Part model, mm, in its own coordinate system. Round coordinates to 2 decimals unless told otherwise and drop trailing zeros. Write each loop counter-clockwise with the first axis right and the second up, starting at its lowest first coordinate (ties: lowest second). Pieces come first, ordered by that corner, then holes. Notation, with made-up numbers: M 20.5,76.25 L 60.5,76.25 A21 cw 60.5,98.25 Z; hole C 14,17 d1. An arc over 180 degrees is marked long. One line per question, with ' | ' between items. Start each with the question number.
1) Saw through at B-B (z = 77.5). List the corners of the cut face in (x, y).
2) Drop flat-ended pins along their axis: pin 1 Ø12 at (x, y) = (9, -44.5) entering from -Z; pin 2 Ø10 at (y, z) = (-64, 26.5) entering from -X; pin 3 Ø4 at (x, y) = (9.5, -52.5) entering from +Z; pin 4 Ø1 at (x, y) = (21.5, -11.5) entering from +Z. Give the stop position or say it passes through.
3) Saw through at C-C (x = -17). List the corners of the cut face in (y, z), plus the area to 3 significant figures.
4) Saw through at A-A (y = -67.5). List the corners of the cut face in (x, z).
5) Saw through at D-D (z = 46.5). List the corners of the cut face in (x, y) (3 decimals).
6) Wall check: probe 1 along Y at (x, z) = (-20.5, 24.5); probe 2 along X at (y, z) = (-26.5, 19); probe 3 along Z at (x, y) = (26, -23). Give the ranges that are in metal, low to high. Write a range as [from, to].
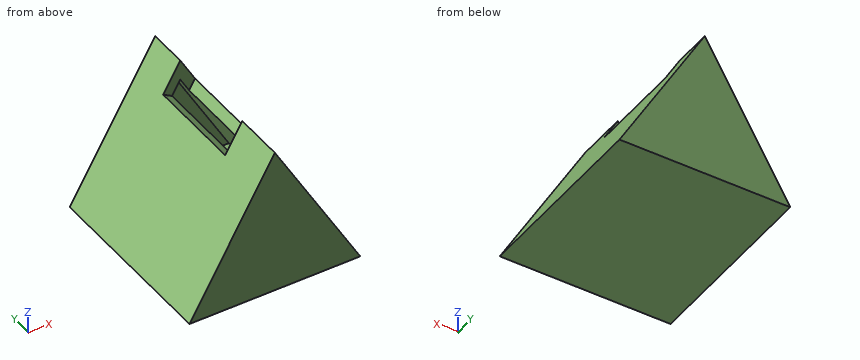
```python
from build123d import *

# Parameters (mm, degrees)
F1_DEPTH = 100
F3_DEPTH = 5
F5_DEPTH = 5
F6_W     = 56.985039264
F6_H     = 20
F7_DEPTH = 15


with BuildPart() as f1:
    # F0 (on Front) → F1 (new body)
    with BuildSketch(Plane.XZ):
        Polygon((0, 86.6025403784), (-50, 0), (50, 0), align=None)
        Polygon((40, 5.3205080757), (-40, 5.3205080757), (0, 74.6025403784), align=None, mode=Mode.SUBTRACT)
    extrude(amount=F1_DEPTH)

    # F2 (on face) → F3 (join)
    with BuildSketch(Plane.XZ.offset(100)):
        Polygon((-50, 0), (50, 0), (0, 86.6025403784), align=None)
        Polygon((0, 74.6025403784), (40, 5.3205080757), (-40, 5.3205080757), align=None, mode=Mode.SUBTRACT)
        Polygon((-40, 5.3205080757), (40, 5.3205080757), (0, 74.6025403784), align=None)
    extrude(amount=F3_DEPTH)

    # F4 (on face) → F5 (join)
    with BuildSketch(Plane(origin=(0, 0, 0), x_dir=(-1, 0, 0), z_dir=(0, 1, 0))):
        Polygon((0, 86.6025403784), (-50, 0), (50, 0), align=None)
        Polygon((0, 74.6025403784), (40, 5.3205080757), (-40, 5.3205080757), align=None, mode=Mode.SUBTRACT)
        Polygon((-40, 5.3205080757), (40, 5.3205080757), (0, 74.6025403784), align=None)
    extrude(amount=F5_DEPTH)

    # F6 (on face) → F7 (cut)
    with BuildSketch(Plane(origin=(-37.5, 0, 21.6506350946), x_dir=(0, -1, 0), z_dir=(-0.8660254038, 0, 0.5))):
        with Locations((46.5483199805, 65)):
            Rectangle(F6_W, F6_H)
    extrude(amount=-F7_DEPTH, mode=Mode.SUBTRACT)


solid = f1.part
```
Answer key:
1) outline: M -5.26,-105 L 5.26,-105 L 5.26,-75.04 L -5.26,-75.04 Z; M -5.26,-18.06 L 5.26,-18.06 L 5.26,5 L -5.26,5 Z
2) pin 1: stops at z = 0 | pin 2: stops at x = -37.59 | pin 3: stops at z = 71.6 | pin 4: stops at z = 50.23
3) outline: M -105,0 L 5,0 L 5,57.16 L -105,57.16 Z; hole M -100,5.32 L 0,5.32 L 0,45.16 L -100,45.16 Z | area: 2,300 mm2
4) outline: M -50,0 L 50,0 L 8.66,71.6 L 5.2,65.6 L 40,5.32 L -40,5.32 L -4.8,66.28 L -10,69.28 Z
5) outline: M -23.153,-105 L 23.153,-105 L 23.153,5 L -23.153,5 Z; hole M -16.225,-100 L 16.225,-100 L 16.225,0 L -16.225,0 Z
6) probe 1: y = [-105, -100], [0, 5] | probe 2: x = [-39.03, -32.1], [32.1, 39.03] | probe 3: z = [0, 5.32], [29.57, 41.57]
